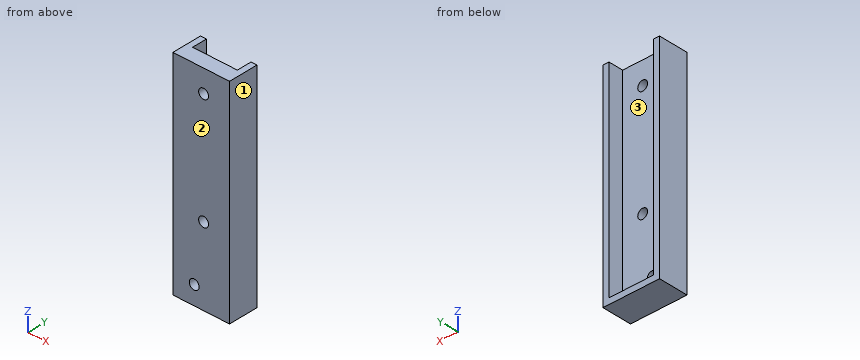
Autodesk Inventor part; units mm, degrees
ref_plane "YZ Plane" through (0, 0, 0) normal (1, 0, 0) x (0, 1, 0)
ref_plane "XZ Plane" through (0, 0, 0) normal (0, 1, 0) x (-1, 0, 0)
ref_plane "XY Plane" through (0, 0, 0) normal (0, 0, 1) x (1, 0, 0)
sketch "Sketch1" plane through (0, 0, 0) normal (0, 1, 0) x (-1, 0, 0)
  line L0 (0, 0) -> (19.177, 0)
  line L1 (19.177, 0) -> (19.177, -88.9)
  line L2 (19.177, -88.9) -> (0, -88.9)
  line L3 (0, -88.9) -> (0, 0)
  line L4 (0, -88.9) -> (0, -91.44)
  line L5 (0, -91.44) -> (19.177, -91.44)
  line L6 (19.177, -91.44) -> (19.177, -88.9)
  line L7 (19.177, 0) -> (21.717, 0)
  line L8 (21.717, 0) -> (21.717, -91.44)
  line L9 (21.717, -91.44) -> (19.177, -91.44)
  line L10 (0, -91.44) -> (-2.54, -91.44)
  line L11 (-2.54, -91.44) -> (-2.54, 0)
  line L12 (-2.54, 0) -> (0, 0)
  dimension "d0" = 19.177
  dimension "d1" = 88.9
  dimension "d2" = 2.54
  dimension "d8" = 2.54
  dimension "d9" = 2.54
extrude "Extrusion1" add sketch "Sketch1" along normal blind 6.35
sketch "Sketch4" plane through (0, 6.35, 0) normal (0, 1, 0) x (1, 0, 0)
  line L0 (-21.717, 0) -> (2.54, 0)
  line L1 (-21.717, 0) -> (-19.177, 0)
  line L2 (2.54, 91.44) -> (-21.717, 91.44)
  line L3 (-21.717, 0) -> (-21.717, 91.44)
  line L4 (-21.717, 91.44) -> (2.54, 91.44)
  line L5 (2.54, 91.44) -> (2.54, 0)
  line L6 (0, 0) -> (0, 88.9)
  line L7 (0, 88.9) -> (-19.177, 88.9)
  line L8 (-19.177, 88.9) -> (-19.177, 0)
  line L9 (-19.177, 0) -> (-21.717, 0)
  dimension "d12" = 2.54
  dimension "d13" = 88.9
extrude "Extrusion3" add sketch "Sketch4" along normal blind 6.35 contours L3 L2 L5 L0 L6 L7 L8
sketch "Sketch5" plane through (0, 6.35, 0) normal (0, 1, 0) x (1, 0, 0)
  line L0 (-19.177, 88.9) -> (0, 88.9)
  line L1 (-19.177, 88.9) -> (-12.6238, 88.9)
  line L2 (-12.6238, 88.9) -> (-12.6238, 83.3882)
  circle A0 centre (-12.6238, 83.3882) radius 2.1082
  line L3 (-12.6238, 83.3882) -> (-8.5852, 83.3882)
  line L4 (-8.5852, 83.3882) -> (-8.5852, 57.9882)
  circle A1 centre (-8.5852, 57.9882) radius 2.1082
  line L5 (-8.5852, 57.9882) -> (-8.5852, 9.7282)
  circle A2 centre (-8.5852, 9.7282) radius 2.1082
  point P0 (0, 0)
  dimension "d16" = 6.5532
  dimension "d17" = 5.5118
  dimension "d18" = 4.2164
  dimension "d19" = 4.0386
  dimension "d20" = 25.4
  dimension "d21" = 4.2164
  dimension "d22" = 48.26
  dimension "d23" = 4.2164
extrude "Extrusion4" cut sketch "Sketch5" against normal blind 6.35
properties part number "wing hole drill"
The listing builds one solid part. Answer for the finished solid, in the listing's coordinates (mm). Face numbers are marked on the shaded views. Round coordinates to 2 decimals unless told otherwise and drop trailing zeros. Write each loop counter-clockwise with the first axis right and the second up, starting at its lowest first coordinate (ties: lowest second). Pieces come first, ordered by that corner, then holes. Notation, with made-up numbers: (-6.5, 69.25) -> (41.5, 69.25) arc R14 ccw to (41.5, 90.25) -> close; hole circle Ø5 at (89, 23.25). An arc over 180 degrees is marked (long way). Use CSV: the item, a comma, the result in double quotes. Start each with the question number.
(1) Consider L1, parallel to X at y = 7.25, z = -21.5; L2, parallel to Z at x = -10, y = 1.25; L3, parallel to Y at x = -12.25, z = -34.5. Determine where each line is inside the solid, lowest interval first. Write a range as from..to.
(2) The mould has two halves that part along X. Classify the marked faces 1, 2 and 3: released by +X, released by -X, zero draft, split by the parting line, or undercut.
(3) Section B-B on y = 10.25 is taken. Give the vertices of the cut face in (x, z).
(4) This flat-tipped pin is pushed along its axis until it touches: pin 1 (1 mm diameter, centred on x = -6, y = 7.5, fed in from +Z). Where does it stop, or does it pass through?
(5) Section C-C on z = -6 is taken. Give the vertices of the cut face in (x, y), then the cut area to 3 significant figures.
(6) Section D-D on y = 1.75 is taken. Give the vertices of the cut face in (x, z), then the cut area to 3 significant figures.
(7) Section A-A on x = -11.75 is taken. Give the vertices of the cut face in (y, z).
A:
1,L1,"x = -21.72..-19.18, 0..2.54"
1,L2,"z = -91.44..-59.55, -56.43..-11.29, -8.17..0"
1,L3,"y = 0..6.35"
2,face 1,"released by +X"
2,face 2,"zero draft"
2,face 3,"undercut"
3,outline,"(-21.72, -91.44) -> (2.54, -91.44) -> (2.54, 0) -> (0, 0) -> (0, -88.9) -> (-19.18, -88.9) -> (-19.18, 0) -> (-21.72, 0) -> close"
4,pin 1,"stops at z = -88.9"
5,outline,"(-21.72, 0) -> (2.54, 0) -> (2.54, 12.7) -> (0, 12.7) -> (0, 6.35) -> (-19.18, 6.35) -> (-19.18, 12.7) -> (-21.72, 12.7) -> close"
5,area,"186 mm²"
6,outline,"(-21.72, -91.44) -> (2.54, -91.44) -> (2.54, 0) -> (-21.72, 0) -> close; hole circle Ø4.22 at (-12.62, -83.39); hole circle Ø4.22 at (-8.59, -57.99); hole circle Ø4.22 at (-8.59, -9.73)"
6,area,"2,180 mm²"
7,outline,"(0, -91.44) -> (12.7, -91.44) -> (12.7, -88.9) -> (6.35, -88.9) -> (6.35, -85.31) -> (0, -85.31) -> close; (0, -81.47) -> (6.35, -81.47) -> (6.35, 0) -> (0, 0) -> close"
